```python
from build123d import *

# Parameters (mm, degrees)
SKETCH1_W                                     = 25.4
SKETCH1_H                                     = 6.35
EXTRUDE1_DEPTH                                = 58.42
CSK_FOR_1_4_FLAT_HEAD_MACHINE_SCREW1_AT_COUNT = 2
CSK_FOR_1_4_FLAT_HEAD_MACHINE_SCREW1_AT_PITCH = 45.72
F_3_8_0_375_DIAMETER_HOLE1_D                  = 9.525


with BuildPart() as part:
    # Sketch1 → Extrude1 (new body)
    with BuildSketch(Plane.XY):
        Rectangle(SKETCH1_W, SKETCH1_H)
    extrude(amount=EXTRUDE1_DEPTH)

    # Sketch3 → CSK for 1/4 Flat Head Machine Screw1 (revolve, cut)
    with BuildSketch(Plane(origin=(0, 3.175, 6.35), x_dir=(0, 0, 1), z_dir=(1, 0, 0))):
        Polygon((0, 0), (0, 6.35), (3.2639, 6.35), (3.2639, 3.652419693), (6.4389, 0), align=None)
    csk_for_1_4_flat_head_machine_screw1 = revolve(axis=Axis((0, 9.525, 6.35), (0, -1, 0)), mode=Mode.SUBTRACT)

    # CSK for 1/4 Flat Head Machine Screw1 at: CSK for 1/4 Flat Head Machine Screw1 ×2
    with Locations(*[(0, 0, i * CSK_FOR_1_4_FLAT_HEAD_MACHINE_SCREW1_AT_PITCH) for i in range(1, CSK_FOR_1_4_FLAT_HEAD_MACHINE_SCREW1_AT_COUNT)]):
        add(csk_for_1_4_flat_head_machine_screw1, mode=Mode.SUBTRACT)

    # 3/8 (0.375) Diameter Hole1 (through all)
    with Locations(Plane(origin=(0, 3.175, 29.21), x_dir=(0, 0, 1), z_dir=(0, 1, 0))):
        with Locations((0, 0)):
            Hole(F_3_8_0_375_DIAMETER_HOLE1_D / 2)


solid = part.part
```
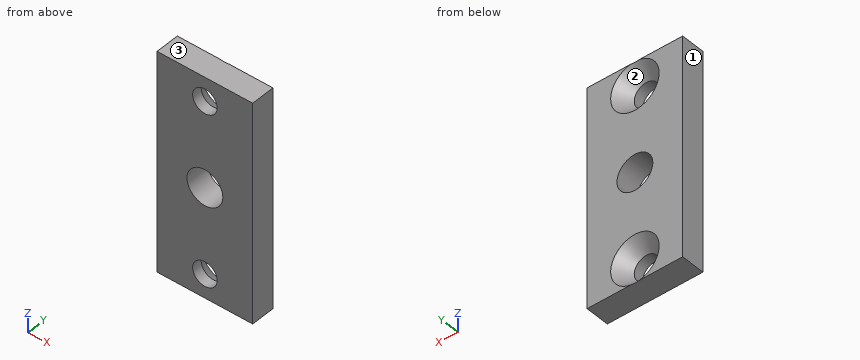
Geometry: final body of the model. Coordinates: model frame, mm. Face numbers are marked on the shaded views. Give positions to 0.01 mm unless a question says otherwise; leave off trailing zeros. Write each loop counter-clockwise with the first axis right and the second up, starting at its lowest first coordinate (ties: lowest second). Pieces come first, ordered by that corner, then holes.
1. Section query C-C, the plane x = 0. Return loops of the section in (y, z) (1 decimal).
2. Draft query along X for the marked faces 1, 2 and 3. Return one class per face: released by +X, released by -X, zero draft, split by the parting line, or undercut.
3. Section query A-A, the plane z = 6.35. Return loops of the section in (x, y) (3 decimals), then the cut area to 3 significant figures.
4. Pin query (flat end, axial travel): P1, Ø8.5, axis at x = 0, z = 6.35, coming from the +Y side; P2, Ø10.5, axis at x = 0, z = 52.07, coming from the +Y side. Return the tip coordinate at first contact, or that it passes through.
5. Line query: probe 1 along Z at (x, y) = (-3, 0.25); probe 2 along X at (y, z) = (-1, 29.21); probe 3 along Z at (x, y) = (-0.75, -2). Output: solid intervals per line, ascending.
6. Section query B-B, the plane y = -1.5. Count the separate pieces of the cut face and the enclosed holes in it, then the cut area to 3 significant figures.
7. Section query D-D, the plane z = 29.21. Return loops of the section in (x, y) (1 decimal), then the cut area to 3 significant figures.
Computed:
1. outline: (-3.2, 0) - (3.1, 0) - (-0.5, 3.1) - (-3.2, 3.1) - close; (-3.2, 9.6) - (-0.5, 9.6) - (3.2, 12.8) - (3.2, 24.4) - (-3.2, 24.4) - close; (-3.2, 34) - (3.2, 34) - (3.2, 45.6) - (-0.5, 48.8) - (-3.2, 48.8) - close; (-3.2, 55.3) - (-0.5, 55.3) - (3.1, 58.4) - (-3.2, 58.4) - close
2. face 1: released by -X
2. face 2: undercut
2. face 3: zero draft
3. outline: (-12.7, -3.175) - (-3.264, -3.175) - (-3.264, -0.477) - (-6.439, 3.175) - (-12.7, 3.175) - close; (3.264, -3.175) - (12.7, -3.175) - (12.7, 3.175) - (6.439, 3.175) - (3.264, -0.477) - close
3. area: 108 mm2
4. P1: stops at y = 0.66
4. P2: stops at y = 1.81
5. probe 1: z = 0 to 3.86, 8.84 to 25.51, 32.91 to 49.58, 54.56 to 58.42
5. probe 2: x = -12.7 to -4.76, 4.76 to 12.7
5. probe 3: z = 0 to 3.17, 9.53 to 24.51, 33.91 to 48.89, 55.25 to 58.42
6. separate pieces: 1
6. enclosed holes: 3
6. area: 1,350 mm2
7. outline: (-12.7, -3.2) - (-4.8, -3.2) - (-4.8, 3.2) - (-12.7, 3.2) - close; (4.8, -3.2) - (12.7, -3.2) - (12.7, 3.2) - (4.8, 3.2) - close
7. area: 101 mm2
